```python
from build123d import *

# Parameters (mm, degrees)
BOSS_EXTRU_1_DEPTH      = 1
ESQUISSE3_R             = 1.25
ENL_V_MAT_EXTRU_1_DEPTH = 3.45
ENL_V_MAT_EXTRU_2_DEPTH = 3.45
SCALE1_SCALE            = 6.5
CUT_EXTRUDE1_DEPTH      = 86.932976581
CUT_EXTRUDE1_DEPTH_BACK = 86.932976581
SKETCH2_W               = 15
SKETCH2_H               = 25
BOSS_EXTRUDE1_DEPTH     = 7.5
SKETCH3_R               = 2.5
CUT_EXTRUDE3_DEPTH      = 93.395152617


with BuildPart() as part:
    # Esquisse1 → Boss.-Extru.1 (new body)
    with BuildSketch(Plane.XY):
        Polygon((15.875, -11.8), (17.7, -11.8), (17.7, 0), (13.225, 0), (9.275, 0), (0, 0), (0, -11.8), (6.625, -11.8), (6.625, -13.9), (15.875, -13.9), align=None)
    extrude(amount=BOSS_EXTRU_1_DEPTH)

    # Esquisse3 → Enlèv. mat.-Extru.1 (cut)
    with BuildSketch(Plane(origin=(0, 0, 0), x_dir=(-1, 0, 0), z_dir=(0, 0, -1))):
        with Locations((-11.25, -8)):
            Circle(ESQUISSE3_R)
    extrude(amount=-ENL_V_MAT_EXTRU_1_DEPTH, mode=Mode.SUBTRACT)

    # Esquisse5 → Enlèv. mat.-Extru.2 (cut)
    with BuildSketch(Plane(origin=(0, 0, 0), x_dir=(-1, 0, 0), z_dir=(0, 0, -1))):
        with BuildLine():
            ThreePointArc((-6.662011173, -5.012361547), (-11.25, -2.525), (-15.837988827, -5.012361547))
            ThreePointArc((-15.837988827, -5.012361547), (-15.545687389, -6.396037763), (-14.162011173, -6.103736324))
            ThreePointArc((-14.162011173, -6.103736324), (-11.25, -4.525), (-8.337988827, -6.103736324))
            ThreePointArc((-8.337988827, -6.103736324), (-6.954312611, -6.396037763), (-6.662011173, -5.012361547))
        make_face()
    extrude(amount=-ENL_V_MAT_EXTRU_2_DEPTH, mode=Mode.SUBTRACT)


with BuildPart() as part_1:
    # Scale1: scaled about (8.774004249, -6.668318819, 0.5)
    add(part.part.scale(SCALE1_SCALE).moved(Location((-48.25702337, 36.675753504, -2.75))))

    # Sketch1 → Cut-Extrude1 (cut, two sides: drawn at the far end of the back side and taken through both)
    with BuildSketch(Plane(origin=(0, 0, -2.75), x_dir=(-1, 0, 0), z_dir=(0, 0, -1)).offset(-CUT_EXTRUDE1_DEPTH_BACK)):
        Polygon((-66.79297663, -27.824246495), (17.05702337, -27.824246495), (17.05702337, 36.675753505), (48.25702337, 36.675753505), (48.25702337, -27.824246495), (48.25702337, -58.098552113), (-66.79297663, -58.098552113), align=None)
    extrude(amount=CUT_EXTRUDE1_DEPTH + CUT_EXTRUDE1_DEPTH_BACK, mode=Mode.SUBTRACT)

    # Sketch2 → Boss-Extrude1 (add)
    with BuildSketch(Plane.XZ.offset(27.824246495)):
        with Locations((-9.55702337, 16.25)):
            Rectangle(SKETCH2_W, SKETCH2_H)
        with Locations((59.29297663, 16.25)):
            Rectangle(SKETCH2_W, SKETCH2_H)
    extrude(amount=-BOSS_EXTRUDE1_DEPTH)

    # Sketch3 → Cut-Extrude3 (cut, through all)
    with BuildSketch(Plane(origin=(0, -20.324246495, 0), x_dir=(1, 0, 0), z_dir=(0, 1, 0))):
        with Locations(Location((-9.55702337, -18.75, 0), (0, 0, 270))):
            Circle(SKETCH3_R)
        with Locations(Location((59.29297663, -18.75, 0), (0, 0, 90))):
            Circle(SKETCH3_R)
    extrude(amount=-CUT_EXTRUDE3_DEPTH, mode=Mode.SUBTRACT)


solid = part_1.part
```
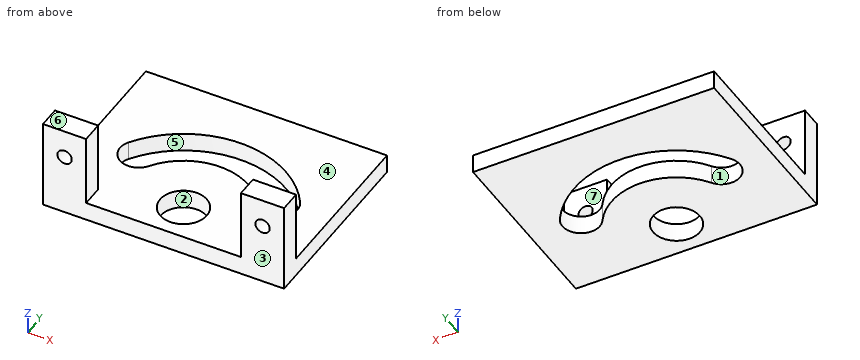
Model file for the job. Use its own axes, mm. Face numbers are marked on the shaded views. A direction names the side the tool comes from. Coordinates: 2 decimals unless noted, no trailing zeros. Loops run counter-clockwise (first coordinate to the right, second up) from the corner with the lowest first, then second, coordinate; pieces in that order, holes last. Notation, with made-up numbers: (-17.75, 41.25) - (28.25, 41.25) arc R4 cw to (28.25, 47.25) - close; hole circle Ø8 at (-35.75, 7). An arc over 180 degrees is marked (long way). Write item = value, one per line. Start each with the question number.
Item 1: Saw through at A-A, the plane z = 18.75. List the corners of the cut face in (x, y).
Item 2: Drop flat-ended pins along their axis: pin 1 Ø4.5 at (x, z) = (-6, 14) entering from +Y; pin 2 Ø12 at (x, y) = (57, -10.5) entering from +Z; pin 3 Ø3 at (x, z) = (59.29, 18.75) entering from +Y; pin 4 Ø6 at (x, y) = (11.5, 3) entering from -Z. Give the stop position or say it passes through.
Item 3: Saw through at D-D, the plane x = 49. List the corners of the cut face in (y, z), then the cut area to 3 significant figures.
Item 4: Saw through at B-B, the plane y = -10. List the corners of the cut face in (x, z), then the cut area to 3 significant figures.
Item 5: Pull direction Y, two halves, no side cores. Call the marked faces 1, 2, 3 and 4: +Y half, -Y half, draft (parallel to the pull), parting line (faces both ways), or undercut.
Item 6: 3-axis set-ups, long thin cutter, end or side, ignore diameter. For the marked faces 5, 6 and 7: which of +Z, -Z, +X, -X, +Y, -Y reach the whole face in a straight line?
Item 7: Saw through at C-C, the plane z = 2. State how many separate pieces and enclosed holes the cut face has, then the cut area to 3 significant figures.
Item 8: Wall check: probe 1 along X at (y, z) = (-25, 18.75); probe 2 along X at (y, z) = (-21.5, 13.5); probe 3 along X at (y, z) = (-22, 18). Give the ranges that are in metal, low to high. Write a range as [from, to].
Answers:
q1.outline = (-17.06, -27.82) - (-12.06, -27.82) - (-12.06, -20.32) - (-17.06, -20.32) - close; (-7.06, -27.82) - (-2.06, -27.82) - (-2.06, -20.32) - (-7.06, -20.32) - close; (51.79, -27.82) - (56.79, -27.82) - (56.79, -20.32) - (51.79, -20.32) - close; (61.79, -27.82) - (66.79, -27.82) - (66.79, -20.32) - (61.79, -20.32) - close
q2.pin_1 = -20.32
q2.pin_2 = 3.75
q2.pin_3 = through
q2.pin_4 = -2.75
q3.outline = (-27.82, -2.75) - (-5.95, -2.75) - (-5.95, 3.75) - (-27.82, 3.75) - close; (10.83, -2.75) - (36.68, -2.75) - (36.68, 3.75) - (10.83, 3.75) - close
q3.area = 310 mm2
q4.outline = (-17.06, -2.75) - (18.73, -2.75) - (18.73, 3.75) - (-17.06, 3.75) - close; (31.01, -2.75) - (66.79, -2.75) - (66.79, 3.75) - (31.01, 3.75) - close
q4.area = 465 mm2
q5.face_1 = undercut
q5.face_2 = undercut
q5.face_3 = -Y half
q5.face_4 = draft
q6.face_5 = +Z, -Z
q6.face_6 = +Z, +X, -X, +Y, -Y
q6.face_7 = +Z, +X, -X, +Y
q7.separate_pieces = 1
q7.enclosed_holes = 2
q7.area = 4,320 mm2
q8.probe_1 = [-17.06, -12.06], [-7.06, -2.06], [51.79, 56.79], [61.79, 66.79]
q8.probe_2 = [-17.06, -2.06], [51.79, 66.79]
q8.probe_3 = [-17.06, -11.94], [-7.17, -2.06], [51.79, 56.91], [61.68, 66.79]
